from build123d import *

# Parameters (mm, degrees)
F0_W     = 30
F0_H     = 46
F0_R     = 8.5
F1_DEPTH = 2
F2_W     = 10
F2_H     = 2
F3_DEPTH = 46
F4_R     = 1.6
F5_DEPTH = 25
F6_R     = 1
F7_R     = 2
F8_R     = 5
F9_R     = 5


with BuildPart() as f1:
    # F0 (on Right) → F1 (new body)
    with BuildSketch(Plane.YZ):
        with Locations((15, 23)):
            Rectangle(F0_W, F0_H)
        with Locations((19.5, 10)):
            Circle(F0_R, mode=Mode.SUBTRACT)
        with Locations((19.5, 36)):
            Circle(F0_R, mode=Mode.SUBTRACT)
    extrude(amount=F1_DEPTH)

    # F2 (on face) → F3 (join)
    with BuildSketch(Plane.XY.offset(46)):
        with Locations((5, 1)):
            Rectangle(F2_W, F2_H)
    extrude(amount=-F3_DEPTH)

    # F4 (on face) → F5 (cut)
    with BuildSketch(Plane.XZ):
        with Locations((6, 30.1)):
            Circle(F4_R)
        with Locations((6, 15.9)):
            Circle(F4_R)
    extrude(amount=-F5_DEPTH, mode=Mode.SUBTRACT)

    # F6
    f6_edges = [f1.edges().sort_by_distance(p)[0] for p in [
        (0, 0, 23),
    ]]
    fillet(f6_edges, radius=F6_R)

    # F7
    f7_edges = [f1.edges().sort_by_distance(p)[0] for p in [
        (2, 2, 23),
    ]]
    fillet(f7_edges, radius=F7_R)

    # F8
    f8_edges = [f1.edges().sort_by_distance(p)[0] for p in [
        (1, 30, 46),
    ]]
    fillet(f8_edges, radius=F8_R)

    # F9
    f9_edges = [f1.edges().sort_by_distance(p)[0] for p in [
        (1, 30, 0),
        (10, 1, 46),
        (10, 1, 0),
    ]]
    fillet(f9_edges, radius=F9_R)


solid = f1.part
For this review, take the finished solid that the model builds, in its own axes (mm). A direction names the side the tool comes from. Give positions to 0.01 mm unless a question says otherwise; leave off trailing zeros. Loops run counter-clockwise (first coordinate to the right, second up) from the corner with the lowest first, then second, coordinate; pieces in that order, holes last. Notation, with made-up numbers: M 62.5,-25.5 L 112.5,-25.5 A6 cw 112.5,-15.5 Z; hole C -24.75,65.25 d6. An arc over 180 degrees is marked long. Answer as a JSON object with one key per item and string values. Group by question number.
Q1. For probe 1 along Z at (x, y) = (0.75, 19.5); probe 2 along Z at (x, y) = (6, 1.5); probe 3 along X at (y, z) = (6, 14.5), list the stretches that pass through material, from the lowest coordinate up. Write a range as [from, to].
Q2. Add section A-A on z = 10. Give the boundary of the cut face in (x, y).
Q3. Mouldability with a two-part tool opening along X and no side actions: class faces 3 (the flat face through (1, 12, 46)), 4 (the flat face through (10, 1, 23)), 5 (the cylindrical face through (5.792, 0.986, 31.686)) as +X half, -X half, draft (parallel to the pull), parting line (faces both ways), or undercut.
Q4. Add section D-D on z = 29. Give the boundary of the cut face in (x, y), and give its area (3 significant figures).
Q5. Tool access review of faces 1 (the flat face through (7, 2, 23)), 2 (the cylindrical face through (1, 29, 2)): name each direction out of +Z, -Z, +X, -X, +Y, -Y from which nothing blocks a thin tool from reaching the whole face with its end or side.
Q6. Add section C-C on x = 6. Give the boundary of the cut face in (y, z).
Q7. Insertion check: P1, Ø13, axis at y = 21, z = 29.5, coming from the +X side; P2, Ø12, axis at y = 9.5, z = 16.5, coming from the +X side; P3, Ø1.8, axis at x = 8.5, z = 32.5, coming from the +Y side. Each pin has a flat end and moves straight along its axis. Give the tip position at first contact, or say it passes through.
Q8. Add section B-B on y = 19.5. Give the boundary of the cut face in (x, z).
Checked values:
{
 "1": {"probe 1": "[0, 1.5], [18.5, 27.5], [44.5, 46]", "probe 2": "[0.1, 14.3], [17.5, 28.5], [31.7, 45.9]", "probe 3": "[0, 2]"},
 "2": {"outline": "M 0,1 A1 ccw 1,0 L 10,0 L 10,2 L 4,2 A2 cw 2,4 L 2,11 L 0,11 Z; M 0,28 L 2,28 L 2,30 L 0,30 Z"},
 "3": {"face 3": "draft", "face 4": "+X half", "face 5": "undercut"},
 "4": {"outline": "M 0,1 A1 ccw 1,0 L 4.84,0 L 4.84,2 L 4,2 A2 cw 2,4 L 2,14.68 L 0,14.68 Z; M 0,24.32 L 2,24.32 L 2,30 L 0,30 Z; M 7.16,0 L 10,0 L 10,2 L 7.16,2 Z", "area": "52.7 mm²"},
 "5": {"face 1": "+Z, -Z, +X, +Y", "face 2": "-Z, +X, -X, +Y"},
 "6": {"outline": "M 0,0.1 L 2,0.1 L 2,14.3 L 0,14.3 Z; M 0,17.5 L 2,17.5 L 2,28.5 L 0,28.5 Z; M 0,31.7 L 2,31.7 L 2,45.9 L 0,45.9 Z"},
 "7": {"P1": "x = 2", "P2": "x = 2.06", "P3": "y = 2"},
 "8": {"outline": "M 0,0 L 2,0 L 2,1.5 L 0,1.5 Z; M 0,18.5 L 2,18.5 L 2,27.5 L 0,27.5 Z; M 0,44.5 L 2,44.5 L 2,46 L 0,46 Z"}
}
